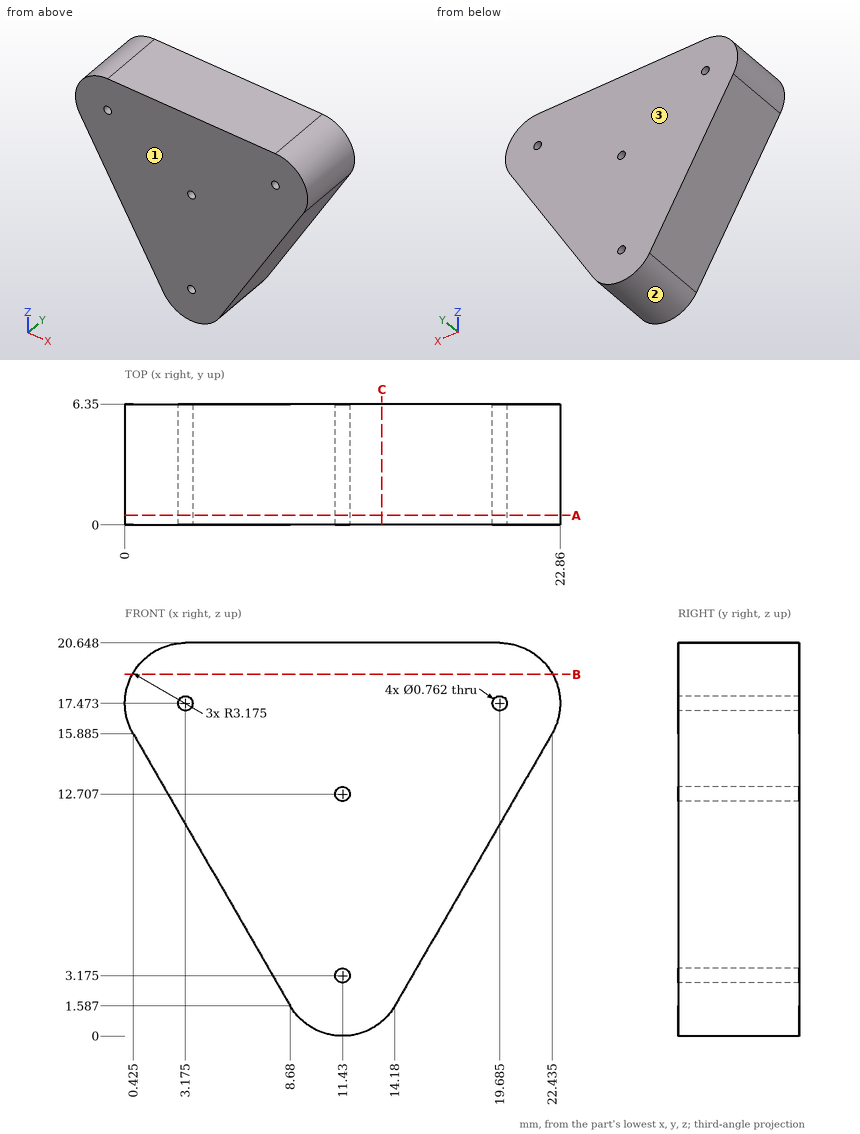
Verification items for this drawing (mm, ordinates from the low corner). Give positions to 0.01 mm unless a question says otherwise; leave off trailing zeros. Loops run counter-clockwise (first coordinate to the right, second up) from the corner with the lowest first, then second, coordinate; pieces in that order, holes last. Notation, with made-up numbers: M 44,12.5 L 65,12.5 A7 cw 65,21.5 Z; hole C -14.5,-1 d5. An arc over 180 degrees is marked long. Answer as a JSON object with one key per item and string values. Group by question number.
Item 1: Sectioned sample at A-A on y = 0.5. Give the number of separate pieces and of enclosed holes in the cut face, plus the area to 3 significant figures.
Item 2: Gauge pin test, flat ends, axial feed: pin 1 (3 mm diameter, centred on y = 1, z = 4.5, fed in from +X); pin 2 (1 mm diameter, centred on y = 2, z = 10.5, fed in from -X) (1 decimal). Record the tip position at first contact, or that the pin passes through.
Item 3: Sectioned sample at B-B on z = 19. Record the boundary of the cut face in (x, y).
Item 4: Material ranges on L1, parallel to X at y = 4, z = 17.5 (1 decimal); L2, parallel to X at y = 4.5, z = 3.25 (1 decimal); L3, parallel to X at y = 5.75, z = 14.25, recorded low to high.
Item 5: Mould release check, pull along Y, two halves, no side actions. Record for the marked faces 1, 2 and 3: pulls with the +Y half, pulls with the -Y half, needs draft (parallel to the pull), parting line crosses it, or undercut.
Item 6: Sectioned sample at C-C on x = 13.5. Record the boundary of the cut face in (y, z), plus the area to 3 significant figures.
Findings below:
{
 "1": {"separate pieces": "1", "enclosed holes": "4", "area": "305 mm2"},
 "2": {"pin 1": "x = 16.73", "pin 2": "x = 3.2"},
 "3": {"outline": "M 0.39,0 L 22.47,0 L 22.47,6.35 L 0.39,6.35 Z"},
 "4": {"L1": "0 to 2.8, 3.6 to 19.3, 20.1 to 22.9", "L2": "7.7 to 11.1, 11.8 to 15.1", "L3": "1.37 to 21.49"},
 "5": {"face 1": "pulls with the -Y half", "face 2": "needs draft", "face 3": "pulls with the +Y half"},
 "6": {"outline": "M 0,0.77 L 6.35,0.77 L 6.35,20.65 L 0,20.65 Z", "area": "126 mm2"}
}
